CAD build for the part. Positions are in the model's coordinates, mm. A direction names the side the tool comes from. Give positions to 0.01 mm unless a question says otherwise; leave off trailing zeros. Write each loop counter-clockwise with the first axis right and the second up, starting at its lowest first coordinate (ties: lowest second). Pieces come first, ordered by that corner, then holes. Notation, with made-up numbers: (18, 48) -> (76, 48) arc R32 cw to (76, 80) -> close; hole circle Ø10 at (-3.75, 46). An arc over 180 degrees is marked (long way). Answer as a JSON object with one key per item and string values.
```python
from build123d import *

# Parameters (mm, degrees)
SKETCH1_R                = 200
BOSS_EXTRUDE1_DEPTH      = 15
BOSS_EXTRUDE2_DEPTH      = 200
CUT_EXTRUDE1_DEPTH       = 286.087705803
CUT_EXTRUDE1_DEPTH_BACK  = 286.087705803
SKETCH3_R                = 85
CUT_EXTRUDE2_DEPTH       = 451.079120005
CUT_EXTRUDE2_DEPTH_BACK  = 451.079120005
SKETCH4_R                = 11
CUT_EXTRUDE3_DEPTH       = 451.079120105
CUT_EXTRUDE3_DEPTH_BACK  = 110
CUT_EXTRUDE4_DEPTH       = 110
BOSS_EXTRUDE3_DEPTH      = 200
CUT_EXTRUDE5_DEPTH       = 286.087705815
CUT_EXTRUDE5_DEPTH_BACK  = 286.087705815
SKETCH7_OUTSIDE_W        = 515.59
SKETCH7_OUTSIDE_H        = 515.59
SKETCH7_OUTSIDE_R        = 200
SKETCH9_R                = 4
BOSS_EXTRUDE4_DEPTH      = 220
CUT_EXTRUDE6_DEPTH       = 190
SKETCH11_R               = 3
CUT_EXTRUDE7_DEPTH       = 486.974499745
CUT_EXTRUDE8_DEPTH       = 302.61434707
CUT_EXTRUDE8_DEPTH_BACK  = 302.61434707
BOSS_EXTRUDE5_DEPTH      = 150
CUT_EXTRUDE9_DEPTH       = 262.287608345
CUT_EXTRUDE9_DEPTH_BACK  = 262.287608345
CUT_EXTRUDE10_DEPTH      = 259.795285906
CUT_EXTRUDE10_DEPTH_BACK = 259.795285906
SKETCH18_R               = 85
CUT_EXTRUDE11_START      = -15
CUT_EXTRUDE11_DEPTH      = 35
SKETCH20_R               = 2.75
CUT_EXTRUDE12_DEPTH      = 268.341007469
SKETCH21_W               = 30
SKETCH21_H               = 5
BOSS_EXTRUDE6_DEPTH      = 37
SKETCH22_R               = 0.95
CUT_EXTRUDE13_DEPTH      = 10
CUT_EXTRUDE14_DEPTH      = 3
LPATTERN1_COUNT          = 3
LPATTERN1_PITCH          = 30
CUT_EXTRUDE15_DEPTH      = 3
LPATTERN2_COUNT          = 3
LPATTERN2_PITCH          = 30
SKETCH25_R               = 3
CUT_EXTRUDE16_DEPTH      = 30


# Read off the part's stored shape, not the designer's step: Cut-Extrude11
with BuildPart() as part:
    # Sketch1 → Boss-Extrude1 (new body)
    with BuildSketch(Plane(origin=(0, 0, 0), x_dir=(1, 0, 0), z_dir=(0, 1, 0))):
        with Locations(Location((0, 0, 0), (0, 0, 270))):
            Circle(SKETCH1_R)
    extrude(amount=BOSS_EXTRUDE1_DEPTH)

    # Sketch2 → Boss-Extrude2 (add, symmetric)
    with BuildSketch(Plane.XY):
        Polygon((-25, 50.707142143), (25, 50.707142143), (60, 15), (-60, 15), align=None)
    extrude(amount=BOSS_EXTRUDE2_DEPTH, both=True)

    # Sketch3 → Cut-Extrude1 (cut, two sides: drawn at the far end of the back side and taken through both)
    with BuildSketch(Plane(origin=(0, 15, 0), x_dir=(1, 0, 0), z_dir=(0, 1, 0)).offset(-CUT_EXTRUDE1_DEPTH_BACK)):
        with Locations(Location((0, 0, 0), (0, 0, 270))):
            Circle(SKETCH3_R)
    extrude(amount=CUT_EXTRUDE1_DEPTH + CUT_EXTRUDE1_DEPTH_BACK, mode=Mode.SUBTRACT)

    # Sketch4 → Cut-Extrude2 (cut, two sides: drawn at the far end of the back side and taken through both)
    with BuildSketch(Plane(origin=(0, 0, -200), x_dir=(-1, 0, 0), z_dir=(0, 0, -1)).offset(-CUT_EXTRUDE2_DEPTH_BACK)):
        with Locations((0, 29)):
            Circle(SKETCH4_R)
    extrude(amount=CUT_EXTRUDE2_DEPTH + CUT_EXTRUDE2_DEPTH_BACK, mode=Mode.SUBTRACT)

    # Sketch5 → Cut-Extrude3 (cut, two sides: drawn at the far end of the back side and taken through both)
    with BuildSketch(Plane.XY.offset(200).offset(-CUT_EXTRUDE3_DEPTH_BACK)):
        Polygon((-25, 50.707142143), (25, 50.707142143), (50.198039412, 25), (25, 25), (25, 15), (-25, 15), (-25, 25), (-50.198039412, 25), align=None)
    extrude(amount=CUT_EXTRUDE3_DEPTH + CUT_EXTRUDE3_DEPTH_BACK, mode=Mode.SUBTRACT)

    # Sketch6 → Cut-Extrude4 (cut)
    with BuildSketch(Plane(origin=(0, 0, -200), x_dir=(-1, 0, 0), z_dir=(0, 0, -1))):
        Polygon((-25, 50.707142143), (25, 50.707142143), (50.198039412, 25), (25, 25), (25, 15), (-25, 15), (-25, 25), (-50.198039412, 25), align=None)
    extrude(amount=-CUT_EXTRUDE4_DEPTH, mode=Mode.SUBTRACT)

    # Sketch8 → Boss-Extrude3 (add, symmetric)
    with BuildSketch(Plane(origin=(0, 0, 0), x_dir=(0, 0, -1), z_dir=(1, 0, 0))):
        Polygon((0, 15), (-20, 15), (-10, 35.712315177), (10, 35.712315177), (20, 15), align=None)
    extrude(amount=BOSS_EXTRUDE3_DEPTH, both=True)

    # Sketch7 outside → Cut-Extrude5 (cut, two sides: drawn at the far end of the back side and taken through both)
    with BuildSketch(Plane(origin=(0, 15, 0), x_dir=(1, 0, 0), z_dir=(0, 1, 0)).offset(-CUT_EXTRUDE5_DEPTH_BACK)):
        Rectangle(SKETCH7_OUTSIDE_W, SKETCH7_OUTSIDE_H)
        with Locations(Location((0, 0, 0), (0, 0, 97.180755781))):
            Circle(SKETCH7_OUTSIDE_R, mode=Mode.SUBTRACT)
    extrude(amount=CUT_EXTRUDE5_DEPTH + CUT_EXTRUDE5_DEPTH_BACK, mode=Mode.SUBTRACT)

    # Sketch9 → Boss-Extrude4 (add, symmetric)
    with BuildSketch(Plane(origin=(0, 0, 0), x_dir=(0, 0, -1), z_dir=(1, 0, 0))):
        with Locations(Location((0, 29, 0), (0, 0, 180))):
            Circle(SKETCH9_R)
    extrude(amount=BOSS_EXTRUDE4_DEPTH, both=True)

    # Sketch10 → Cut-Extrude6 (cut, symmetric)
    with BuildSketch(Plane(origin=(0, 0, 0), x_dir=(0, 0, -1), z_dir=(1, 0, 0))):
        Polygon((-20, 15), (20, 15), (10, 35.712315177), (-10, 35.712315177), align=None)
    extrude(amount=CUT_EXTRUDE6_DEPTH, both=True, mode=Mode.SUBTRACT)

    # Sketch11 → Cut-Extrude7 (cut, through all)
    with BuildSketch(Plane.ZY.offset(220)):
        with Locations((0, 29)):
            Circle(SKETCH11_R)
    extrude(amount=-CUT_EXTRUDE7_DEPTH, mode=Mode.SUBTRACT)

    # Sketch14 → Cut-Extrude8 (cut, two sides: drawn at the far end of the back side and taken through both)
    with BuildSketch(Plane(origin=(0, 0, 0), x_dir=(1, 0, 0), z_dir=(0, 1, 0)).offset(-CUT_EXTRUDE8_DEPTH_BACK)):
        Polygon((-80, 28.722813233), (-80, 204.683452683), (-270.013244013, 28.722813233), (-103.583737584, -216.10995611), (187.046893047, -216.10995611), (266.535612536, 150.034958035), (80, 209.154693155), (80, 28.722813233), align=None)
    extrude(amount=CUT_EXTRUDE8_DEPTH + CUT_EXTRUDE8_DEPTH_BACK, mode=Mode.SUBTRACT)

    # Sketch16 → Boss-Extrude5 (add, symmetric)
    with BuildSketch(Plane(origin=(0, 0, -90), x_dir=(-1, 0, 0), z_dir=(0, 0, -1))):
        Polygon((-80, 15), (-80, 35), (-70, 35), (-70, 25), (-61, 15), (-61, 0), (-80, 0), (-80, 4.5), (-90, 4.5), (-90, 10.5), (-80, 10.5), align=None)
        Polygon((80, 15), (80, 35), (70, 35), (70, 25), (61, 15), (61, 0), (80, 0), (80, 4.5), (90, 4.5), (90, 10.5), (80, 10.5), align=None)
    extrude(amount=BOSS_EXTRUDE5_DEPTH, both=True)

    # Sketch17 → Cut-Extrude9 (cut, two sides: drawn at the far end of the back side and taken through both)
    with BuildSketch(Plane(origin=(0, 0, 0), x_dir=(1, 0, 0), z_dir=(0, 1, 0)).offset(-CUT_EXTRUDE9_DEPTH_BACK)):
        Polygon((-80, 28.722813233), (-99.608008808, 28.722813233), (-99.608008808, -74.271563426), (112.245925984, -74.271563426), (112.245925984, 0), (109.222119936, 28.722813233), (80, 28.722813233), align=None)
    extrude(amount=CUT_EXTRUDE9_DEPTH + CUT_EXTRUDE9_DEPTH_BACK, mode=Mode.SUBTRACT)

    # Sketch18 → Cut-Extrude10 (cut, two sides: drawn at the far end of the back side and taken through both)
    with BuildSketch(Plane(origin=(0, 15, 0), x_dir=(1, 0, 0), z_dir=(0, 1, 0)).offset(-CUT_EXTRUDE10_DEPTH_BACK)):
        Circle(SKETCH18_R)
    extrude(amount=CUT_EXTRUDE10_DEPTH + CUT_EXTRUDE10_DEPTH_BACK, mode=Mode.SUBTRACT)

    # Cut-Extrude11 outline → Cut-Extrude11 (cut)
    with BuildSketch(Plane(origin=(0, 15, 0), x_dir=(1, 0, 0), z_dir=(0, 1, 0)).offset(CUT_EXTRUDE11_START)):
        with BuildLine():
            Line((61, 240), (61, 190.470470152))
            ThreePointArc((61, 190.470470152), (75.732708439, 185.106879593), (90, 178.605710995))
            Line((90, 178.605710995), (90, 240))
            Line((90, 240), (61, 240))
        make_face()
        with BuildLine():
            Line((-61, 190.470470152), (-61, 240))
            Line((-61, 240), (-90, 240))
            Line((-90, 240), (-90, 178.605710995))
            ThreePointArc((-90, 178.605710995), (-75.732708439, 185.106879593), (-61, 190.470470152))
        make_face()
    extrude(amount=CUT_EXTRUDE11_DEPTH, mode=Mode.SUBTRACT)

    # Sketch20 → Cut-Extrude12 (cut, through all)
    with BuildSketch(Plane.ZY.offset(80)):
        with Locations((-163.303027798, 30)):
            Circle(SKETCH20_R)
        with Locations((-103.303027798, 30)):
            Circle(SKETCH20_R)
        with Locations((-133.303027798, 30)):
            Circle(SKETCH20_R)
    extrude(amount=-CUT_EXTRUDE12_DEPTH, mode=Mode.SUBTRACT)

    # Sketch21 → Boss-Extrude6 (add)
    with BuildSketch(Plane(origin=(0, 15, 0), x_dir=(1, 0, 0), z_dir=(0, 1, 0))):
        with Locations((0, 114.6)):
            Rectangle(SKETCH21_W, SKETCH21_H)
    extrude(amount=BOSS_EXTRUDE6_DEPTH)

    # Sketch22 → Cut-Extrude13 (cut)
    with BuildSketch(Plane(origin=(0, 0, -117.1), x_dir=(-1, 0, 0), z_dir=(0, 0, -1))):
        with Locations((-8.93, 23.49)):
            Circle(SKETCH22_R)
        with Locations((8.93, 23.49)):
            Circle(SKETCH22_R)
        with Locations((8.93, 34.49)):
            Circle(SKETCH22_R)
        with Locations((-8.93, 34.49)):
            Circle(SKETCH22_R)
    extrude(amount=-CUT_EXTRUDE13_DEPTH, mode=Mode.SUBTRACT)

    # Sketch23 → Cut-Extrude14 (cut)
    with BuildSketch(Plane(origin=(-70, 0, 0), x_dir=(0, 0, -1), z_dir=(1, 0, 0))):
        Polygon((103.303027798, 34.1), (105.668027798, 34.1), (108.035163902, 30), (105.668027798, 25.9), (103.303027798, 25.9), (100.938027798, 25.9), (98.570891695, 30), (100.938027798, 34.1), align=None)
    cut_extrude14 = extrude(amount=-CUT_EXTRUDE14_DEPTH, mode=Mode.SUBTRACT)

    # LPattern1: Cut-Extrude14 ×3
    with Locations(*[(0, 0, -i * LPATTERN1_PITCH) for i in range(1, LPATTERN1_COUNT)]):
        add(cut_extrude14, mode=Mode.SUBTRACT)

    # Sketch24 → Cut-Extrude15 (cut)
    with BuildSketch(Plane.ZY.offset(-70)):
        Polygon((-163.303027798, 34.09260032), (-160.933027798, 34.09260032), (-158.568027798, 29.99630016), (-160.933027798, 25.9), (-163.303027798, 25.9), (-165.673027798, 25.9), (-168.038027798, 29.99630016), (-165.673027798, 34.09260032), align=None)
    cut_extrude15 = extrude(amount=-CUT_EXTRUDE15_DEPTH, mode=Mode.SUBTRACT)

    # LPattern2: Cut-Extrude15 ×3
    with Locations(*[(0, 0, i * LPATTERN2_PITCH) for i in range(1, LPATTERN2_COUNT)]):
        add(cut_extrude15, mode=Mode.SUBTRACT)

    # Sketch25 → Cut-Extrude16 (cut)
    with BuildSketch(Plane(origin=(0, 15, 0), x_dir=(1, 0, 0), z_dir=(0, 1, 0))):
        with Locations(Location((-18.923887281, 105.579050088, 0), (0, 0, 270))):
            Circle(SKETCH25_R)
    extrude(amount=-CUT_EXTRUDE16_DEPTH, mode=Mode.SUBTRACT)


solid = part.part
```
1) 3-axis set-ups, long thin cutter, end or side, ignore diameter. For faces 1 (the flat face through (-73, 32, -131)), 2 (the flat face through (-25, 20, -145)), 3 (the flat face through (0, 33, -112.1)), 4 (the flat face through (-50.52, 24.67, -125.97)), 5 (the flat face through (-85, 10.5, -107)): which of +Z, -Z, +X, -X, +Y, -Y reach the whole face in a straight line?
Model answer:
{"face 1": "none", "face 2": "-Z, +Y", "face 3": "+Y", "face 4": "+Z, -Z, +Y", "face 5": "+Z, -Z, -X, +Y"}
2) Pin check, flat tips, straight feed: pin 1 (5 mm diameter, centred on y = 31.5, z = -87, fed in from -X); pin 2 (2.5 mm diameter, centred on y = 28.5, z = -135, fed in from +X); pin 3 (8 mm diameter, centred on x = -46.5, z = -135.5, fed in from +Y); pin 4 (2.5 mm diameter, centred on y = 31, z = -162.5, fed in from +X). Stop position of each tip, or through.
Model answer:
{"pin 1": "stops at x = -80", "pin 2": "stops at x = 80", "pin 3": "stops at y = 25", "pin 4": "passes through"}
3) Slice it at B-B (y = 43.5). List the corners of the cut face in (x, z), then the cut area to 3 significant figures.
Model answer:
{"outline": "(-32.06, -90) -> (32.06, -90) -> (32.06, -78.72) arc R85 cw to (-32.06, -78.72) -> close; (-15, -117.1) -> (15, -117.1) -> (15, -112.1) -> (-15, -112.1) -> close", "area": "603 mm2"}
4) Slice it at A-A (z = -87.5). List the corners of the cut face in (x, y), then the cut area to 3 significant figures.
Model answer:
{"outline": "(-90, 4.5) -> (-80, 4.5) -> (-80, 0) -> (80, 0) -> (80, 4.5) -> (90, 4.5) -> (90, 10.5) -> (80, 10.5) -> (80, 35) -> (70, 35) -> (70, 25) -> (61, 15) -> (60, 15) -> (25, 50.71) -> (-25, 50.71) -> (-60, 15) -> (-61, 15) -> (-70, 25) -> (-70, 35) -> (-80, 35) -> (-80, 10.5) -> (-90, 10.5) -> close; hole circle Ø22 at (0, 29)", "area": "5,660 mm2"}
5) Slice it at C-C (z = -39.5). List the corners of the cut face in (x, y).
Model answer:
{"outline": "(-90, 4.5) -> (-80, 4.5) -> (-80, 0) -> (-75.26, 0) -> (-75.26, 35) -> (-80, 35) -> (-80, 10.5) -> (-90, 10.5) -> close; (75.26, 0) -> (80, 0) -> (80, 4.5) -> (90, 4.5) -> (90, 10.5) -> (80, 10.5) -> (80, 35) -> (75.26, 35) -> close"}
6) Wall check: probe 1 along Y at (x, z) = (-8.93, -113.3); probe 2 along Y at (x, z) = (0, -85.5); probe 3 along X at (y, z) = (29, -88.05). Give the ranges that are in metal, low to high.
Model answer:
{"probe 1": "y = 0 to 22.54, 24.44 to 33.54, 35.44 to 52", "probe 2": "y = 0 to 18, 40 to 50.71", "probe 3": "x = -80 to -70, -46.28 to -11, 11 to 46.28, 70 to 80"}
7) Slice it at D-D (z = -121). List the corners of the cut face in (x, y), then the cut area to 3 significant figures.
Model answer:
{"outline": "(-90, 4.5) -> (-80, 4.5) -> (-80, 0) -> (80, 0) -> (80, 4.5) -> (90, 4.5) -> (90, 10.5) -> (80, 10.5) -> (80, 35) -> (70, 35) -> (70, 25) -> (61, 15) -> (60, 15) -> (50.2, 25) -> (25, 25) -> (25, 15) -> (-25, 15) -> (-25, 25) -> (-50.2, 25) -> (-60, 15) -> (-61, 15) -> (-70, 25) -> (-70, 35) -> (-80, 35) -> (-80, 10.5) -> (-90, 10.5) -> close", "area": "3,610 mm2"}
8) Mould opens along X. For faces 6 (the flat face through (0, 52, -115)), 7 (the flat face through (90, 7, -103)), 8 (the flat face through (0, 33, -117.1)) say: released by +X, released by -X, zero draft, split by the parting line, or undercut.
Model answer:
{"face 6": "zero draft", "face 7": "released by +X", "face 8": "undercut"}
